Autodesk Inventor part; units mm, degrees
ref_plane "YZ Plane" through (0, 0, 0) normal (1, 0, 0) x (0, 1, 0)
ref_plane "XZ Plane" through (0, 0, 0) normal (0, 1, 0) x (-1, 0, 0)
ref_plane "XY Plane" through (0, 0, 0) normal (0, 0, 1) x (1, 0, 0)
sketch "Sketch1" plane through (0, 0, 0) normal (0, 0, 1) x (1, 0, 0)
  line L0 (17, -13) -> (-17, -13)
  line L1 (-17, -13) -> (-17, 13)
  line L2 (-17, 13) -> (17, 13)
  line L3 (17, 13) -> (17, -13)
  line L4 (17, -13) -> (-17, 13) construction
  line L5 (-17, -13) -> (17, 13) construction
  point P0 (0, 0)
  dimension "d0" = 34
  dimension "d1" = 26
extrude "Extrusion1" add sketch "Sketch1" along normal blind 3
sketch "Sketch3" plane through (0, 0, 3) normal (0, 0, 1) x (1, 0, 0)
  point P0 (0, 0)
  point P1 (-8, 0)
  point P2 (8, 0)
  point P3 (0, 6)
  point P4 (0, -6)
  dimension "d4" = 12
  dimension "d5" = 16
  dimension "d6" = 8
  dimension "d7" = 6
hole "Hole1" at (-8, 0, 3) at (8, 0, 3) direction (0, 0, -1) diameter 1.5 end through all
sketch "Sketch4" plane through (0, 0, 3) normal (0, 0, 1) x (1, 0, 0)
  point P0 (0, 0)
  point P1 (0, 0)
hole "Hole2" at (0, 0, 3) direction (0, 0, -1) diameter 8 end through all
properties part number "Firewall" material "Plywood"
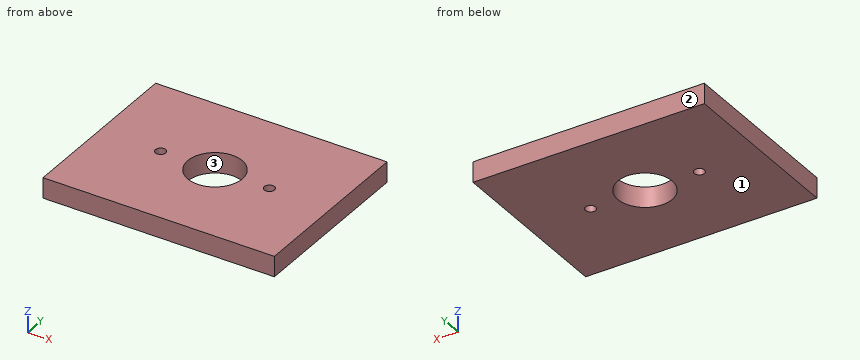
Part model, mm, in its own coordinate system. Face numbers are marked on the shaded views. Round coordinates to 2 decimals unless told otherwise and drop trailing zeros. Order: outer loops, then holes, each group sorted by start corner. A loop starts at its lowest first (then second) coordinate and runs counter-clockwise, first axis right, second up. Notation, with made-up numbers: M 59.5,-25.5 L 71.5,-25.5 A19 ccw 71.5,-21.5 Z; hole C 15.25,75 d7. An arc over 180 degrees is marked long. Put each result on its own line as item: value. Start each with the question number.
1. Slice it at B-B on y = 0. List the corners of the cut face in (x, z), then the cut area to 3 significant figures.
2. Drill centre lines: probe 1 along X at (y, z) = (0, 2.35); probe 2 along Y at (x, z) = (8, 2.15); probe 3 along Y at (x, z) = (0, 1.6). Where is each one in solid material? Low to high. Write a range as [from, to].
3. Slice it at A-A on x = 8. List the corners of the cut face in (y, z).
4. Slice it at D-D on x = -3. List the corners of the cut face in (y, z).
5. Drop a flat-ended pin along its axis: pin 1 (1.4 mm diameter, centred on x = -8, y = 0, fed in from +Z). Give the stop position or say it passes through.
6. Slice it at C-C on z = 2.4. List the corners of the cut face in (x, y).
7. Two-plate mould, pull along Y, no slides. Class the marked faces 1, 2 and 3: +Y half, -Y half, draft (parallel to the pull), parting line (faces both ways), or undercut.
Findings:
1. outline: M -17,0 L -8.75,0 L -8.75,3 L -17,3 Z; M -7.25,0 L -4,0 L -4,3 L -7.25,3 Z; M 4,0 L 7.25,0 L 7.25,3 L 4,3 Z; M 8.75,0 L 17,0 L 17,3 L 8.75,3 Z
1. area: 69.0 mm2
2. probe 1: [-17, -8.75], [-7.25, -4], [4, 7.25], [8.75, 17]
2. probe 2: [-13, -0.75], [0.75, 13]
2. probe 3: [-13, -4], [4, 13]
3. outline: M -13,0 L -0.75,0 L -0.75,3 L -13,3 Z; M 0.75,0 L 13,0 L 13,3 L 0.75,3 Z
4. outline: M -13,0 L -2.65,0 L -2.65,3 L -13,3 Z; M 2.65,0 L 13,0 L 13,3 L 2.65,3 Z
5. pin 1: through
6. outline: M -17,-13 L 17,-13 L 17,13 L -17,13 Z; hole C -8,0 d1.5; hole C 0,0 d8; hole C 8,0 d1.5
7. face 1: draft
7. face 2: +Y half
7. face 3: undercut
